Part model, mm, in its own coordinate system. A direction names the side the tool comes from. Coordinates: 2 decimals unless noted, no trailing zeros. Order: outer loops, then holes, each group sorted by start corner. A loop starts at its lowest first (then second) coordinate and runs counter-clockwise, first axis right, second up.
Autodesk Inventor part; units mm, degrees
ref_plane "YZ Plane" through (0, 0, 0) normal (1, 0, 0) x (0, 1, 0)
ref_plane "XZ Plane" through (0, 0, 0) normal (0, 1, 0) x (-1, 0, 0)
ref_plane "XY Plane" through (0, 0, 0) normal (0, 0, 1) x (1, 0, 0)
sketch "Sketch1" plane through (0, 0, 0) normal (0, 0, 1) x (1, 0, 0)
  circle A0 centre (10, 32.5) radius 36
  line L0 (22, 0.6881) -> (22, 4)
  line L1 (22, 4) -> (20, 4)
  line L2 (20, 4) -> (20, 0)
  line L3 (16.7, 4) -> (15, 4)
  line L4 (22, 64.3119) -> (22, 61)
  line L5 (22, 61) -> (20, 61)
  line L6 (20, 61) -> (20, 65)
  line L7 (16.7, 61) -> (15, 61)
  line L8 (16.7, 61) -> (14.7, 61)
  line L9 (14.7, 61) -> (14.7, 66.1736)
  line L10 (16.7, 65.8333) -> (16.7, 61)
  line L11 (16.7, 4) -> (14.7, 4)
  line L12 (14.7, 4) -> (14.7, -1.1736)
  line L13 (16.7, -0.8333) -> (16.7, 4)
  arc A1 (16.7, -0.8333) -> (20, 0.0038) centre (10, 32.5) ccw
  arc A2 (14.7, 66.1736) -> (14.7, -1.1736) centre (10, 32.5) ccw
  arc A3 (22, 0.6881) -> (22, 64.3119) centre (10, 32.5) ccw
  arc A4 (20, 64.9962) -> (16.7, 65.8333) centre (10, 32.5) ccw
  point P0 (0, 0)
extrude "Extrusion1" add sketch "Sketch1" along normal blind 140
sketch "Sketch2" plane through (10, 32.5, 140) normal (0, 0, 1) x (1, 0, 0)
  circle A0 centre (0, 0) radius 36
  point P0 (-10, -32.5)
extrude "Extrusion2" add sketch "Sketch2" along normal blind 3
sketch "Sketch3" plane through (10, 32.5, 143) normal (0, 0, 1) x (1, 0, 0)
  circle A0 centre (0, 0) radius 3.85
  arc A1 (-2.15, -1.2757) -> (-2.15, 1.2757) centre (0, 0) ccw
  line L0 (-2.15, 0) -> (-2.15, 1.2757)
  line L1 (-2.15, 0) -> (-2.15, -1.2757)
  point P0 (-10, -32.5)
  dimension "d14" = 7.7
  dimension "d15" = 5
extrude "Extrusion3" add sketch "Sketch3" along normal blind 30
sketch "Sketch4" plane through (10, 32.5, 143) normal (0, 0, 1) x (1, 0, 0)
  circle A0 centre (0, 0) radius 6
  point P0 (-10, -32.5)
  dimension "d19" = 12
extrude "Extrusion4" add sketch "Sketch4" along normal blind 15
sketch "Sketch5" plane through (10, 32.5, 0) normal (0, 0, -1) x (-1, 0, 0)
  line L0 (-22.5, 36.2326) -> (-22.5, -36.2326)
  line L1 (-22.5, -36.2326) -> (22.5, -36.2326)
  line L2 (22.5, -36.2326) -> (22.5, 36.2326)
  line L3 (22.5, 36.2326) -> (-22.5, 36.2326)
  line L4 (-22.5, 36.2326) -> (22.5, -36.2326) construction
  line L5 (-22.5, -36.2326) -> (22.5, 36.2326) construction
  circle A0 centre (0, 0) radius 36
  point P0 (10, -32.5)
  point P1 (-22.5, -28.1025)
  point P2 (-22.5, 28.1025)
  point P3 (22.5, 28.1025)
  point P4 (22.5, -28.1025)
  dimension "d22" = 45
  dimension "d25" = 72.4652
extrude "Extrusion5" cut sketch "Sketch5" against normal blind 140 contours L0 A0 | A0 L2
properties part number "Casing"
(1) Probe line 1 (Y direction, x = 10, z = 167.25); line 2 (X direction, y = 2, z = 99); line 3 (Z direction, x = 24, y = 54). List the from-to ranges inside material, lowest first.
(2) Tool access for faces 1 (the face through (12, 67, 0)), 2 (the face through (20, 2, 69)), 3 (the face through (12.5, 32.59, 165.4)): list every direction of +Z, -Z, +X, -X, +Y, -Y with a clear straight run to the whole face (end or side of a thin tool).
(3) Slice it at C-C, the plane z = 150. Give the cut face in (x, y).
(4) Slice it at D-D, the plane y = 48.5. Give the cut face in (x, z).
(5) Pull direction Y, two halves, no side cores. Call faces 4 (the face through (12.07, 29.254, 165.395)), 5 (the face through (13, 33, 173)), 6 (the face through (27.463, 61.672, 69.02)), 7 (the face through (0.01, 65, 69.02)): +Y half, -Y half, draft (parallel to the pull), parting line (faces both ways), or undercut.
(6) Slice it at B-B, the plane x = 10. Give the cut face in (y, z), then the cut area to 3 significant figures.
(7) Slice it at A-A, the plane z = 79.5. Give the cut face in (x, y).
(8) Drop flat-ended pins along their axis: pin 1 (1 mm diameter, centred on y = 2.5, z = 40, fed in from +X); pin 2 (5 mm diameter, centred on x = 33.5, z = 60.5, fed in from -Y); pin 3 (3 mm diameter, centred on y = 5.5, z = 52, fed in from +X); pin 4 (6 mm diameter, centred on x = -12.5, y = 58.5, fed in from -Z). Give the stop position or say it passes through.
Here are the results:
1. line 1: y = 28.65 to 30, 35 to 36.35
1. line 2: x = -9.12 to -5.03, 14.7 to 16.7, 20 to 22, 25.02 to 29.12
1. line 3: z = 140 to 143
2. face 1: -Z, +X, -X, +Y, -Y
2. face 2: -Z
2. face 3: +Z
3. outline: circle Ø12 at (10, 32.5)
4. outline: (-22.25, 140) - (42.25, 140) - (42.25, 143) - (-22.25, 143) - close
5. face 4: parting line
5. face 5: draft
5. face 6: undercut
5. face 7: undercut
6. outline: (-3.5, 0) - (-1.5, 0) - (-1.5, 140) - (66.5, 140) - (66.5, 0) - (68.5, 0) - (68.5, 143) - (38.5, 143) - (38.5, 158) - (36.35, 158) - (36.35, 173) - (35, 173) - (35, 158) - (30, 158) - (30, 173) - (28.65, 173) - (28.65, 158) - (26.5, 158) - (26.5, 143) - (-3.5, 143) - close
6. area: 996 mm2
7. outline: (-12.5, 4.4) arc R36 ccw to (32.5, 4.4) - (32.5, 7.01) arc R34 cw to (22, 0.69) - (22, 4) - (20, 4) - (20, 0) arc R34.02 cw to (16.7, -0.83) - (16.7, 4) - (14.7, 4) - (14.7, -1.17) arc R34 cw to (-12.5, 7.01) - close; (-12.5, 57.99) arc R34 cw to (14.7, 66.17) - (14.7, 61) - (16.7, 61) - (16.7, 65.83) arc R33.98 cw to (20, 65) - (20, 61) - (22, 61) - (22, 64.31) arc R34 cw to (32.5, 57.99) - (32.5, 60.6) arc R36 ccw to (-12.5, 60.6) - close
8. pin 1: stops at x = 30.63
8. pin 2: stops at y = 3.26
8. pin 3: stops at x = 32.5
8. pin 4: stops at z = 0
